from build123d import *

# Parameters (mm, degrees)
F0_R     = 3.175
F1_DEPTH = 66.675
F2_DEPTH = 25.4
F3_DEPTH = 22.225
F0_R_2   = 1.5875
F4_DEPTH = 3.175
F5_R     = 22.86


with BuildPart() as f1:
    # F0 (on Front) → F1 (new body)
    with BuildSketch(Plane.XZ):
        Polygon((25.4, -25.003125), (0, -25.003125), (-25.4, -25.003125), (-25.4, -34.528125), (-25.4, -44.053125), (25.4, -44.053125), align=None)
        with BuildLine():
            ThreePointArc((-9.525, -34.528125), (-12.7, -37.703125), (-15.875, -34.528125))
            ThreePointArc((-15.875, -34.528125), (-12.7, -31.353125), (-9.525, -34.528125))
        make_face(mode=Mode.SUBTRACT)
        with Locations((12.7, -34.528125)):
            Circle(F0_R, mode=Mode.SUBTRACT)
    extrude(amount=F1_DEPTH)

    # F0 (on Front) → F2 (join)
    with BuildSketch(Plane.XZ):
        with BuildLine():
            Line((-25.4, -25.003125), (0, -25.003125))
            ThreePointArc((0, -25.003125), (-17.6798792384, -17.6798792384), (-25.003125, 0))
            Line((-25.003125, 0), (-25.4, 0))
            Line((-25.4, 0), (-25.4, -25.003125))
        make_face()
        with BuildLine():
            Line((25.4, 0), (25.003125, 0))
            ThreePointArc((25.003125, 0), (17.6798792384, -17.6798792384), (0, -25.003125))
            Line((0, -25.003125), (25.4, -25.003125))
            Line((25.4, -25.003125), (25.4, 0))
        make_face()
    extrude(amount=F2_DEPTH)

    # F0 (on Front) → F3 (cut)
    with BuildSketch(Plane.XZ):
        with BuildLine():
            Line((-25.4, -25.003125), (0, -25.003125))
            ThreePointArc((0, -25.003125), (-17.6798792384, -17.6798792384), (-25.003125, 0))
            Line((-25.003125, 0), (-25.4, 0))
            Line((-25.4, 0), (-25.4, -25.003125))
        make_face()
        with BuildLine():
            Line((25.4, 0), (25.003125, 0))
            ThreePointArc((25.003125, 0), (17.6798792384, -17.6798792384), (0, -25.003125))
            Line((0, -25.003125), (25.4, -25.003125))
            Line((25.4, -25.003125), (25.4, 0))
        make_face()
    extrude(amount=F3_DEPTH, mode=Mode.SUBTRACT)

    # F0 (on Front) → F4 (join)
    with BuildSketch(Plane.XZ):
        with BuildLine():
            ThreePointArc((11.906250128, -20.6222298537), (20.6222299646, -11.906249936), (23.8125, 0))
            ThreePointArc((23.8125, 0), (20.6222299411, 11.9062499767), (11.9062500466, 20.6222299007))
            ThreePointArc((11.9062500466, 20.6222299007), (3.75e-08, 23.8125), (-11.9062499816, 20.6222299383))
            ThreePointArc((-11.9062499816, 20.6222299383), (-20.6222299223, 11.9062500092), (-23.8125, 0))
            ThreePointArc((-23.8125, 0), (-20.622229928, -11.9062499993), (-11.9062500014, -20.6222299268))
            ThreePointArc((-11.9062500014, -20.6222299268), (7.31e-08, -23.8125), (11.906250128, -20.6222298537))
        make_face()
        with BuildLine():
            ThreePointArc((-9.525, -19.2474145991), (-10.3187500007, -20.622229928), (-11.9062500014, -20.6222299268))
            ThreePointArc((-11.9062500014, -20.6222299268), (-11.9062499993, -17.8725992702), (-9.525, -19.2474145991))
        make_face(mode=Mode.SUBTRACT)
        with BuildLine():
            ThreePointArc((12.7, -19.2474145991), (12.4873153655, -20.0411645351), (11.906250128, -20.6222298537))
            ThreePointArc((11.906250128, -20.6222298537), (9.7376846345, -18.4536646631), (12.7, -19.2474145991))
        make_face(mode=Mode.SUBTRACT)
        with BuildLine():
            ThreePointArc((-20.6375, 0), (-22.225, -1.5875), (-23.8125, 0))
            ThreePointArc((-23.8125, 0), (-22.225, 1.5875), (-20.6375, 0))
        make_face(mode=Mode.SUBTRACT)
        with BuildLine():
            ThreePointArc((-9.525, 19.2474145991), (-11.9062500092, 17.8725992759), (-11.9062499816, 20.6222299383))
            ThreePointArc((-11.9062499816, 20.6222299383), (-10.3187499908, 20.6222299223), (-9.525, 19.2474145991))
        make_face(mode=Mode.SUBTRACT)
        with Locations((22.225, 0)):
            Circle(F0_R_2, mode=Mode.SUBTRACT)
        with BuildLine():
            ThreePointArc((12.7, 19.2474145991), (9.737684658, 18.4536646224), (11.9062500466, 20.6222299007))
            ThreePointArc((11.9062500466, 20.6222299007), (12.487315342, 20.0411645758), (12.7, 19.2474145991))
        make_face(mode=Mode.SUBTRACT)
        with BuildLine():
            Line((23.8125, 0), (25.003125, 0))
            ThreePointArc((25.003125, 0), (17.6798792384, 17.6798792384), (0, 25.003125))
            ThreePointArc((0, 25.003125), (-17.6798792384, 17.6798792384), (-25.003125, 0))
            Line((-25.003125, 0), (-23.8125, 0))
            ThreePointArc((-23.8125, 0), (-20.6222299223, 11.9062500092), (-11.9062499816, 20.6222299383))
            ThreePointArc((-11.9062499816, 20.6222299383), (3.75e-08, 23.8125), (11.9062500466, 20.6222299007))
            ThreePointArc((11.9062500466, 20.6222299007), (20.6222299411, 11.9062499767), (23.8125, 0))
        make_face()
        with BuildLine():
            Line((25.4, 0), (25.003125, 0))
            ThreePointArc((25.003125, 0), (17.6798792384, -17.6798792384), (0, -25.003125))
            Line((0, -25.003125), (25.4, -25.003125))
            Line((25.4, -25.003125), (25.4, 0))
        make_face()
        with BuildLine():
            Line((-25.4, -25.003125), (0, -25.003125))
            ThreePointArc((0, -25.003125), (-17.6798792384, -17.6798792384), (-25.003125, 0))
            Line((-25.003125, 0), (-25.4, 0))
            Line((-25.4, 0), (-25.4, -25.003125))
        make_face()
        with BuildLine():
            ThreePointArc((0, 25.003125), (17.6798792384, 17.6798792384), (25.003125, 0))
            Line((25.003125, 0), (25.4, 0))
            Line((25.4, 0), (25.4, 25.003125))
            Line((25.4, 25.003125), (0, 25.003125))
        make_face()
        with BuildLine():
            ThreePointArc((-25.003125, 0), (-17.6798792384, 17.6798792384), (0, 25.003125))
            Line((0, 25.003125), (-25.4, 25.003125))
            Line((-25.4, 25.003125), (-25.4, 0))
            Line((-25.4, 0), (-25.003125, 0))
        make_face()
        with BuildLine():
            ThreePointArc((0, -25.003125), (17.6798792384, -17.6798792384), (25.003125, 0))
            Line((25.003125, 0), (23.8125, 0))
            ThreePointArc((23.8125, 0), (20.6222299646, -11.906249936), (11.906250128, -20.6222298537))
            ThreePointArc((11.906250128, -20.6222298537), (7.31e-08, -23.8125), (-11.9062500014, -20.6222299268))
            ThreePointArc((-11.9062500014, -20.6222299268), (-20.622229928, -11.9062499993), (-23.8125, 0))
            Line((-23.8125, 0), (-25.003125, 0))
            ThreePointArc((-25.003125, 0), (-17.6798792384, -17.6798792384), (0, -25.003125))
        make_face()
    extrude(amount=F4_DEPTH)

    # F5
    f5_edges = [f1.edges().sort_by_distance(p)[0] for p in [
        (25.4, -1.5875, 25.003125),
        (-25.4, -1.5875, 25.003125),
    ]]
    fillet(f5_edges, radius=F5_R)


solid = f1.part
Check sheet for the modelled part. Datum: model origin and axes. Units: mm. A direction names the side the tool comes from. Round coordinates to 2 decimals unless told otherwise and drop trailing zeros. Order: outer loops, then holes, each group sorted by start corner. A loop starts at its lowest first (then second) coordinate and runs counter-clockwise, first axis right, second up.
Q1. Draft check along Y on faces 1 (the face through (0, -2, 25.003)), 2 (the face through (-20, -22.225, -18)), 3 (the face through (0, -13, -25.003)), 4 (the face through (20, -25.4, -19)). Enter one of: pulls with the +Y half, pulls with the -Y half, needs draft (parallel to the pull), parting line crosses it, or undercut.
Filled sheet:
face 1: needs draft
face 2: undercut
face 3: undercut
face 4: pulls with the -Y half
Q2. Cross-section at B-B, the plane y = -18. Enter the section's corners in (x, z) (3 decimals), plus the area to 3 significant figures.
Filled sheet:
outline: (-25.4, -44.053) - (25.4, -44.053) - (25.4, -25.003) - (-25.4, -25.003) - close; hole circle Ø6.35 at (-12.7, -34.528); hole circle Ø6.35 at (12.7, -34.528)
area: 904 mm2
Q3. Depth check by flat-ended pin: P1, Ø2, axis at x = 19.5, y = -51, coming from the +Z side; P2, Ø2, axis at x = 16.5, z = 2, coming from the -Y side (3 decimals); P3, Ø2.5, axis at x = 22.225, z = 0, coming from the -Y side. Enter the tip coordinate at first touch or a pass-through.
Filled sheet:
P1: stops at z = -25
P2: stops at y = -3.175
P3: passes through
Q4. Set-up check for faces 5 (the face through (-18.88, -1.61, 18.13)), 6 (the face through (0, -46, -25.003)), 7 (the face through (20, -22.225, -19)): record each of +Z, -Z, +X, -X, +Y, -Y from which the full face is reachable in a straight line by a thin tool's end or side.
Filled sheet:
face 5: +Z, -X, +Y, -Y
face 6: +Z, +X, -X, -Y
face 7: +Z, +X, -X
Q5. Cross-section at C-C, the plane x = -18. Enter the section's corners in (y, z) (3 decimals).
Filled sheet:
outline: (-66.675, -44.053) - (0, -44.053) - (0, 18.983) - (-3.175, 18.983) - (-3.175, -25.003) - (-22.225, -25.003) - (-22.225, -17.354) - (-25.4, -17.354) - (-25.4, -25.003) - (-66.675, -25.003) - close
Q6. Cross-section at A-A, the plane x = -6. Enter the section's corners in (y, z) (3 decimals).
Filled sheet:
outline: (-66.675, -44.053) - (0, -44.053) - (0, 24.74) - (-3.175, 24.74) - (-3.175, -25.003) - (-22.225, -25.003) - (-22.225, -24.273) - (-25.4, -24.273) - (-25.4, -25.003) - (-66.675, -25.003) - close
Q7. Scan lines: L1, parallel to Z at x = 12.5, y = -31; L2, parallel to Y at x = -10, z = -14 (3 decimals); L3, parallel to X at y = -33, z = -32.5. Record each from-to range of solid material in increasing order.
Filled sheet:
L1: z = -44.05 to -37.7, -31.36 to -25
L2: y = -3.175 to 0
L3: x = -25.4 to -15.14, -10.26 to 10.26, 15.14 to 25.4
